Check sheet for the modelled part. Datum: model origin and axes. Units: mm. A direction names the side the tool comes from. Coordinates: 2 decimals unless noted, no trailing zeros. Write each loop counter-clockwise with the first axis right and the second up, starting at its lowest first coordinate (ties: lowest second). Pieces come first, ordered by that corner, then holes. Notation, with made-up numbers: (20.5, 10) -> (77.5, 10) arc R15 ccw to (77.5, 31) -> close; hole circle Ø9 at (8, -12). An arc over 180 degrees is marked (long way). One line per item, written item: value. Start each with the question number.
1) Sectioned sample at C-C on x = 5.5. Enter the section's corners in (y, z), plus the area to 3 significant figures.
2) Gauge pin test, flat ends, axial feed: P1, Ø3.5, axis at x = 3, y = -4, coming from the +Z side; P2, Ø8, axis at x = 6.5, y = 16, coming from the +Z side; P3, Ø1, axis at x = 39.5, z = 8, coming from the -Y side; P4, Ø5, axis at y = 3, z = 21.5, coming from the -X side. Record the tip position at first contact, or that the pin passes through.
3) Sectioned sample at D-D on y = -4. Enter the section's corners in (x, z), plus the area to 3 significant figures.
4) Scan lines: line 1 along Y through (x, z) = (17.5, 25.75); line 2 along Z through (x, y) = (56.5, -1); line 3 along Y through (x, z) = (49.5, 1.5). Record each from-to range of solid material in increasing order. Write a range as [from, to].
5) Sectioned sample at B-B on z = 21.25. Enter the section's corners in (x, y), plus the area to 3 significant figures.
6) Draft check along X on faces 1 (the flat face through (50.2, -1, 16)), 2 (the flat face through (52.2, 13, 2)), 3 (the flat face through (0, 4, 3)), 4 (the cylindrical face through (55.3, -2.6, 4.6)). Enter one of: +X half, -X half, draft (parallel to the pull), parting line (faces both ways), or undercut.
7) Sectioned sample at A-A on y = 7. Enter the section's corners in (x, z), plus the area to 3 significant figures.
8) Set-up check for faces 5 (the flat face through (3, 13, 2)), 6 (the flat face through (10, 11, 2)), 7 (the flat face through (2, -3.17, 15)), 8 (the flat face through (30, -4, 4)), 9 (the flat face through (7.25, -5, 15)): record each of +Z, -Z, +X, -X, +Y, -Y from which the full face is reachable in a straight line by a thin tool's end or side.
```python
from build123d import *

# Parameters (mm, degrees)
SKETCH1_W             = 10
SKETCH1_H             = 25
BOSS_EXTRUDE1_DEPTH   = 4
BOSS_EXTRUDE1_2_DEPTH = 4
SKETCH1_3_W           = 40.2
SKETCH1_3_H           = 2
BOSS_EXTRUDE2_DEPTH   = 29
SKETCH1_4_W           = 10
SKETCH1_4_H           = 2
BOSS_EXTRUDE3_DEPTH   = 4
FILLET2_R             = 2
SKETCH2_W             = 60.2
SKETCH2_H             = 4
BOSS_EXTRUDE5_DEPTH   = 4.17
SKETCH3_W             = 10
SKETCH3_H             = 3
BOSS_EXTRUDE6_DEPTH   = 20
FILLET3_R             = 2
CUT_EXTRUDE1_DEPTH    = 15


with BuildPart() as part:
    # Sketch1 → Boss-Extrude1 (new body)
    with BuildSketch(Plane.XY):
        with Locations((5, 12.5)):
            Rectangle(SKETCH1_W, SKETCH1_H)
        with BuildLine():
            ThreePointArc((3, 4.75), (5.5, 2.25), (8, 4.75))
            Line((8, 4.75), (8, 20.75))
            ThreePointArc((8, 20.75), (5.5, 23.25), (3, 20.75))
            Line((3, 20.75), (3, 4.75))
        make_face(mode=Mode.SUBTRACT)
    extrude(amount=BOSS_EXTRUDE1_DEPTH)



with BuildPart() as body_2:
    # Sketch1 → Boss-Extrude1 2 (new body)
    with BuildSketch(Plane.XY):
        with Locations((55.2, 12.5)):
            Rectangle(SKETCH1_W, SKETCH1_H)
        with BuildLine():
            Line((57.2, 20.75), (57.2, 4.75))
            ThreePointArc((57.2, 4.75), (54.7, 2.25), (52.2, 4.75))
            Line((52.2, 4.75), (52.2, 20.75))
            ThreePointArc((52.2, 20.75), (54.7, 23.25), (57.2, 20.75))
        make_face(mode=Mode.SUBTRACT)
    extrude(amount=BOSS_EXTRUDE1_2_DEPTH)


with BuildPart() as body_3:
    # Sketch1<3> → Boss-Extrude2 (new body)
    with BuildSketch(Plane.XY):
        with Locations((30.1, -1)):
            Rectangle(SKETCH1_3_W, SKETCH1_3_H)
    extrude(amount=BOSS_EXTRUDE2_DEPTH)


with BuildPart() as part_1:
    add(part.part)

    add(body_2.part)  # Boss-Extrude3 merges body 2

    add(body_3.part)  # Boss-Extrude3 merges body 3
    # Sketch1<4> → Boss-Extrude3 (add)
    with BuildSketch(Plane.XY):
        with Locations((5, -1)):
            Rectangle(SKETCH1_4_W, SKETCH1_4_H)
        with Locations((55.2, -1)):
            Rectangle(SKETCH1_4_W, SKETCH1_4_H)
    extrude(amount=BOSS_EXTRUDE3_DEPTH)

    # Fillet2
    fillet2_edges = [part_1.edges().sort_by_distance(p)[0] for p in [
        (0, 25, 2),
        (10, 25, 2),
        (60.2, 25, 2),
        (50.2, 25, 2),
    ]]
    fillet(fillet2_edges, radius=FILLET2_R)

    # Sketch2 → Boss-Extrude5 (add)
    with BuildSketch(Plane.XZ.offset(2)):
        with Locations((30.1, 2)):
            Rectangle(SKETCH2_W, SKETCH2_H)
    extrude(amount=BOSS_EXTRUDE5_DEPTH)

    # Sketch3 → Boss-Extrude6 (add)
    with BuildSketch(Plane.XY.offset(4)):
        with Locations((5, -4.67)):
            Rectangle(SKETCH3_W, SKETCH3_H)
        with Locations((55.2, -4.67)):
            Rectangle(SKETCH3_W, SKETCH3_H)
    extrude(amount=BOSS_EXTRUDE6_DEPTH)

    # Fillet3
    # the kernel refuses this fillet: 2 mm, written as the material it adds along each edge
    with BuildSketch(Plane(origin=(60.2, -3.17, 4), x_dir=(0, 1, 0), z_dir=(-1, 0, 0)), Plane(origin=(10, -3.17, 4), x_dir=(0, 1, 0), z_dir=(-1, 0, 0))) as fillet3_piece_1:
        with BuildLine():
            CenterArc((FILLET3_R, -FILLET3_R), FILLET3_R, 90, 90)
            Line((0, -FILLET3_R), (0, 0))
            Line((0, 0), (FILLET3_R, 0))
        make_face()
    extrude(amount=10)

    # Sketch4 → Cut-Extrude1 (cut)
    with BuildSketch(Plane(origin=(0, -3.17, 0), x_dir=(1, 0, 0), z_dir=(0, 1, 0))):
        with BuildLine():
            Line((7.25, -20), (7.25, -10))
            ThreePointArc((7.25, -10), (5, -7.75), (2.75, -10))
            Line((2.75, -10), (2.75, -20))
            ThreePointArc((2.75, -20), (5, -22.25), (7.25, -20))
        make_face()
        with BuildLine():
            ThreePointArc((52.95, -10), (55.2, -7.75), (57.45, -10))
            Line((57.45, -10), (57.45, -20))
            ThreePointArc((57.45, -20), (55.2, -22.25), (52.95, -20))
            Line((52.95, -20), (52.95, -10))
        make_face()
    extrude(amount=-CUT_EXTRUDE1_DEPTH, mode=Mode.SUBTRACT)


solid = part_1.part
```
Answers:
1. outline: (-6.17, 0) -> (2.25, 0) -> (2.25, 4) -> (-1.17, 4) arc R2 cw to (-3.17, 6) -> (-3.17, 7.81) -> (-6.17, 7.81) -> close; (-6.17, 22.19) -> (-3.17, 22.19) -> (-3.17, 24) -> (-6.17, 24) -> close; (23.25, 0) -> (25, 0) -> (25, 4) -> (23.25, 4) -> close
1. area: 58.4 mm2
2. P1: stops at z = 24
2. P2: stops at z = 4
2. P3: stops at y = -2
2. P4: passes through
3. outline: (0, 0) -> (60.2, 0) -> (60.2, 24) -> (50.2, 24) -> (50.2, 4) -> (10, 4) -> (10, 24) -> (0, 24) -> close; hole (2.75, 10) arc R2.25 ccw to (7.25, 10) -> (7.25, 20) arc R2.25 ccw to (2.75, 20) -> close; hole (52.95, 10) arc R2.25 ccw to (57.45, 10) -> (57.45, 20) arc R2.25 ccw to (52.95, 20) -> close
3. area: 519 mm2
4. line 1: y = [-2, 0]
4. line 2: z = [0, 4]
4. line 3: y = [-6.17, 0]
5. outline: (0, -6.17) -> (3.13, -6.17) -> (3.13, -3.17) -> (0, -3.17) -> close; (6.87, -6.17) -> (10, -6.17) -> (10, -3.17) -> (6.87, -3.17) -> close; (10, -2) -> (50.2, -2) -> (50.2, 0) -> (10, 0) -> close; (50.2, -6.17) -> (53.33, -6.17) -> (53.33, -3.17) -> (50.2, -3.17) -> close; (57.07, -6.17) -> (60.2, -6.17) -> (60.2, -3.17) -> (57.07, -3.17) -> close
5. area: 118 mm2
6. face 1: +X half
6. face 2: undercut
6. face 3: -X half
6. face 4: draft
7. outline: (0, 0) -> (3, 0) -> (3, 4) -> (0, 4) -> close; (8, 0) -> (10, 0) -> (10, 4) -> (8, 4) -> close; (50.2, 0) -> (52.2, 0) -> (52.2, 4) -> (50.2, 4) -> close; (57.2, 0) -> (60.2, 0) -> (60.2, 4) -> (57.2, 4) -> close
7. area: 40.0 mm2
8. face 5: +Z, -Z
8. face 6: +Z, -Z, +Y
8. face 7: +Z, +X, -X, +Y
8. face 8: +Z, -Y
8. face 9: +Y, -Y
